Geometry check sheet. Reference: the model listing, model coordinates, mm. A direction names the side the tool comes from. Coordinates: 2 decimals unless noted, no trailing zeros. Order: outer loops, then holes, each group sorted by start corner. A loop starts at its lowest first (then second) coordinate and runs counter-clockwise, first axis right, second up. Notation, with made-up numbers: (67, 79) -> (76, 79) arc R25 ccw to (76, 117) -> close; hole circle Ø10 at (85.5, 8). An arc over 180 degrees is marked (long way). Answer as CSV lines item,"result". Start each with the question number.
Autodesk Inventor part; units mm, degrees
ref_plane "YZ Plane" through (0, 0, 0) normal (1, 0, 0) x (0, 1, 0)
ref_plane "XZ Plane" through (0, 0, 0) normal (0, 1, 0) x (-1, 0, 0)
ref_plane "XY Plane" through (0, 0, 0) normal (0, 0, 1) x (1, 0, 0)
sketch "Sketch1" plane through (0, 0, 0) normal (0, 0, 1) x (1, 0, 0)
  line L0 (0, 4) -> (0, 26)
  line L1 (0, 26) -> (10, 26)
  line L2 (10, 26) -> (10, 30)
  line L3 (10, 30) -> (25, 30)
  line L4 (25, 30) -> (25, 26)
  line L5 (25, 26) -> (35, 26)
  line L6 (35, 26) -> (35, 4)
  line L7 (35, 4) -> (25, 4)
  line L8 (25, 4) -> (25, 0)
  line L9 (25, 0) -> (10, 0)
  line L10 (10, 0) -> (10, 4)
  line L11 (0, 4) -> (10, 4)
  point P0 (0, 0)
  dimension "d0" = 22
  dimension "d1" = 10
  dimension "d2" = 4
  dimension "d3" = 15
  dimension "d4" = 10
  dimension "d5" = 22
extrude "Extrusion1" add sketch "Sketch1" along normal blind 4
properties part number "stubbur"
Q1. Sectioned sample at B-B, the plane y = 2.5. Record the cut outline in (x, z), then the cut area to 3 significant figures.
Q2. Go/stop test with flat-tipped pins: pin 1 Ø1.5 at (x, z) = (9, 3.5) entering from +Y; pin 2 Ø2 at (x, z) = (4, 2.5) entering from -Y; pin 3 Ø1.2 at (y, z) = (28.5, 2) entering from -X. Record where each tip stops, or that it passes through.
Q3. Release check for a two-part mould opening along Z. For faces 1 (the flat face through (17, 15, 0)), 2 (the flat face through (30, 4, 2)), 3 (the flat face through (17, 15, 4)) record: released by +Z, released by -Z, zero draft, split by the parting line, or undercut.
Q4. Thickness scan on L1, parallel to Y at x = 29, z = 3.1; L2, parallel to X at y = 2.25, z = 0.5. Record the ranges inside material, lowest first.
Q5. Access from +Z, -Z, +X, -X, +Y, -Y to the whole of each face (thin tool, end or side, straight path). Record for faces 4 (the flat face through (10, 28, 2)), 5 (the flat face through (25, 2, 2)), 6 (the flat face through (30, 26, 2)).
Q6. Sectioned sample at C-C, the plane x = 26. Record the cut outline in (y, z), then the cut area to 3 significant figures.
Q7. Sectioned sample at A-A, the plane z = 0.8. Record the cut outline in (x, y).
Geometry results:
1,outline,"(10, 0) -> (25, 0) -> (25, 4) -> (10, 4) -> close"
1,area,"60.0 mm^2"
2,pin 1,"stops at y = 26"
2,pin 2,"stops at y = 4"
2,pin 3,"stops at x = 10"
3,face 1,"released by -Z"
3,face 2,"zero draft"
3,face 3,"released by +Z"
4,L1,"y = 4 to 26"
4,L2,"x = 10 to 25"
5,face 4,"+Z, -Z, -X, +Y"
5,face 5,"+Z, -Z, +X, -Y"
5,face 6,"+Z, -Z, +X, +Y"
6,outline,"(4, 0) -> (26, 0) -> (26, 4) -> (4, 4) -> close"
6,area,"88.0 mm^2"
7,outline,"(0, 4) -> (10, 4) -> (10, 0) -> (25, 0) -> (25, 4) -> (35, 4) -> (35, 26) -> (25, 26) -> (25, 30) -> (10, 30) -> (10, 26) -> (0, 26) -> close"
